Geometry check sheet. Reference: the model listing, model coordinates, mm. Round coordinates to 2 decimals unless told otherwise and drop trailing zeros. Write each loop counter-clockwise with the first axis right and the second up, starting at its lowest first coordinate (ties: lowest second). Pieces come first, ordered by that corner, then holes. Notation, with made-up numbers: M 72.5,-6.75 L 76.5,-6.75 A29 ccw 76.5,14.25 Z; hole C 24,-3 d8. An arc over 180 degrees is marked long. Put each result on its own line as item: value. Start each with the question number.
(1) Section check B-B on z = 12.8. Count the separate pieces of the cut face and the enclosed holes in it, then the cut area to 3 significant figures.
(2) Section check C-C on y = 28. Record the cut outline in (x, z) (3 decimals).
(3) Section check A-A on y = -28. Record the cut outline in (x, z) (3 decimals), then the cut area to 3 significant figures.
(4) Gauge pin test, flat ends, axial feed: pin 1 (1 mm diameter, centred on x = 64.5, z = 13.5, fed in from +Y); pin 2 (1 mm diameter, centred on x = 65, z = 13.5, fed in from -Y); pin 3 (7 mm diameter, centred on x = -14.51, y = 86.03, fed in from +Z) (3 decimals); pin 4 (4 mm diameter, centred on x = 19.35, y = 77.48, fed in from +Z). Record the tip position at first contact, or that the pin passes through.
(5) Mould release check, pull along Y, two halves, no side actions. Record for faces 1 (the cylindrical face through (-12.9, -30.1, 13.4)), 2 (the flat face through (7, -35, 13)), 3 (the flat face through (80.144, 66, 13)): pulls with the +Y half, pulls with the -Y half, needs draft (parallel to the pull), parting line crosses it, or undercut.
(6) Material ranges on probe 1 along Y at (x, z) = (-15, 13.1); probe 2 along Y at (x, z) = (53.5, 13.25); probe 3 along X at (y, z) = (-27, 13.2), recorded low to high.
from build123d import *

# Parameters (mm, degrees)
SKETCH1_W                                         = 112.782
SKETCH1_H                                         = 3.175
BOSS_EXTRUDE1_DEPTH                               = 99.75
BOSS_EXTRUDE1_DEPTH_BACK                          = 35
SKETCH2_R                                         = 3.175
CUT_EXTRUDE1_DEPTH                                = 15.975
CUT_EXTRUDE1_DEPTH_BACK                           = 1
M4_CLEARANCE_HOLE1_D                              = 4.3
CSK_FOR_4_FLAT_HEAD_MACHINE_SCREW_100_D           = 2.9464
CSK_FOR_4_FLAT_HEAD_MACHINE_SCREW_100_CSINK_D     = 5.715
CSK_FOR_4_FLAT_HEAD_MACHINE_SCREW_100_CSINK_ANGLE = 100
SKETCH8_R                                         = 3
CUT_EXTRUDE3_DEPTH                                = 3.5
F_6_32_TAPPED_HOLE1_D                             = 2.7051
F_1_4_20_TAPPED_HOLE1_D                           = 5.1054
SKETCH16_R                                        = 2.9972
CUT_EXTRUDE4_DEPTH                                = 4.175


with BuildPart() as part:
    # Sketch1 → Boss-Extrude1 (new body, two sides)
    with BuildSketch(Plane(origin=(0, 0, 0), x_dir=(1, 0, 0), z_dir=(0, 1, 0))) as boss_extrude1_sk:
        with Locations((23.753, -13.3875)):
            Rectangle(SKETCH1_W, SKETCH1_H)
    extrude(amount=BOSS_EXTRUDE1_DEPTH)
    extrude(boss_extrude1_sk.sketch, amount=-BOSS_EXTRUDE1_DEPTH_BACK)

    # Sketch2 → Cut-Extrude1 (cut, two sides)
    with BuildSketch(Plane.XY) as cut_extrude1_sk:
        with Locations((67.816, 68.973813735)):
            Circle(SKETCH2_R)
        with Locations((52.316, 68.973813735)):
            Circle(SKETCH2_R)
        Polygon((48, -35), (80.144, -35), (80.144, 22.487287802), (48, -0.020183306), align=None)
        with BuildLine():
            Line((60.066, 56.550419976), (80.066, 56.550419976))
            ThreePointArc((80.066, 56.550419976), (88.066, 48.550419976), (80.066, 40.550419976))
            Line((80.066, 40.550419976), (60.066, 40.550419976))
            ThreePointArc((60.066, 40.550419976), (52.066, 48.550419976), (60.066, 56.550419976))
        make_face()
        Polygon((43.964687276, 99.75), (80.144, 74.416972504), (80.144, 99.75), align=None)
    extrude(amount=CUT_EXTRUDE1_DEPTH, mode=Mode.SUBTRACT)
    extrude(cut_extrude1_sk.sketch, amount=-CUT_EXTRUDE1_DEPTH_BACK, mode=Mode.SUBTRACT)

    # M4 Clearance Hole1 (through all)
    with Locations(Plane.XY.offset(14.975)):
        with Locations((-13.356, 28), (31.644, 28), (31.644, -28), (-13.356, -28)):
            Hole(M4_CLEARANCE_HOLE1_D / 2)

    # CSK for #4 Flat Head Machine Screw (100)1 (through all)
    with Locations(Plane.XY.offset(14.975)):
        with Locations((19.352, 96.519071488), (28.871071488, 87), (19.352, 77.480928512)):
            CounterSinkHole(CSK_FOR_4_FLAT_HEAD_MACHINE_SCREW_100_D / 2, CSK_FOR_4_FLAT_HEAD_MACHINE_SCREW_100_CSINK_D / 2, counter_sink_angle=CSK_FOR_4_FLAT_HEAD_MACHINE_SCREW_100_CSINK_ANGLE)

    # Sketch8 → Cut-Extrude3 (cut)
    with BuildSketch(Plane.XY.offset(14.975)):
        with Locations((19.352, 87)):
            Circle(SKETCH8_R)
    extrude(amount=-CUT_EXTRUDE3_DEPTH, mode=Mode.SUBTRACT)

    # #6-32 Tapped Hole1 (through all)
    with Locations(Plane.XY.offset(14.975)):
        with Locations((-28.824, -3.758), (-21.077, 4.878), (-28.824, 13.514)):
            Hole(F_6_32_TAPPED_HOLE1_D / 2)

    # 1/4-20 Tapped Hole1 (through all)
    with Locations(Plane.XY.offset(14.975)):
        with Locations((57.526, 13.97), (71.75, 13.97), (71.75, 69.85), (57.526, 69.85)):
            Hole(F_1_4_20_TAPPED_HOLE1_D / 2)

    # Sketch16 → Cut-Extrude4 (cut, through all)
    with BuildSketch(Plane.XY.offset(14.975)):
        with Locations((-14.5061, 86.034)):
            Circle(SKETCH16_R)
    extrude(amount=-CUT_EXTRUDE4_DEPTH, mode=Mode.SUBTRACT)


solid = part.part
Answers follow:
1. separate pieces: 1
1. enclosed holes: 15
1. area: 12,600 mm^2
2. outline: M -32.638,11.8 L -15.506,11.8 L -15.506,14.975 L -32.638,14.975 Z; M -11.206,11.8 L 29.494,11.8 L 29.494,14.975 L -11.206,14.975 Z; M 33.794,11.8 L 80.144,11.8 L 80.144,14.975 L 33.794,14.975 Z
3. outline: M -32.638,11.8 L -15.506,11.8 L -15.506,14.975 L -32.638,14.975 Z; M -11.206,11.8 L 29.494,11.8 L 29.494,14.975 L -11.206,14.975 Z; M 33.794,11.8 L 48,11.8 L 48,14.975 L 33.794,14.975 Z
3. area: 229 mm^2
4. pin 1: stops at y = 85.72
4. pin 2: stops at y = 11.53
4. pin 3: stops at z = 14.975
4. pin 4: stops at z = 14.26
5. face 1: undercut
5. face 2: pulls with the -Y half
5. face 3: needs draft
6. probe 1: y = -35 to -29.39, -26.61 to 26.61, 29.39 to 83.08, 88.99 to 99.75
6. probe 2: y = 3.83 to 43.98, 53.12 to 66.03, 71.92 to 93.07
6. probe 3: x = -32.64 to -15.26, -11.45 to 29.74, 33.55 to 48
